```python
from build123d import *

# Parameters (mm, degrees)
ESQUISSE1_W             = 300
ESQUISSE1_H             = 300
BOSS_EXTRU_1_DEPTH      = 12
ESQUISSE2_W             = 250
ESQUISSE2_H             = 250
BOSS_EXTRU_2_DEPTH      = 50
ENL_V_MAT_EXTRU_1_DEPTH = 10
ENL_V_START             = -5
ESQUISSE4_W             = 55
ESQUISSE4_H             = 43.476241007
ENL_V_MAT_EXTRU_2_DEPTH = 5
ESQUISSE6_W             = 240
ESQUISSE6_H             = 240
ENL_V_MAT_EXTRU_3_DEPTH = 50


with BuildPart() as part:
    # Esquisse1 → Boss.-Extru.1 (new body)
    with BuildSketch(Plane.XY):
        Rectangle(ESQUISSE1_W, ESQUISSE1_H)
    extrude(amount=BOSS_EXTRU_1_DEPTH)

    # Esquisse2 → Boss.-Extru.2 (add)
    with BuildSketch(Plane.XY.offset(12)):
        Rectangle(ESQUISSE2_W, ESQUISSE2_H)
    extrude(amount=BOSS_EXTRU_2_DEPTH)

    # Esquisse3 → Enlèv. mat.-Extru.1 (cut)
    with BuildSketch(Plane(origin=(0, 0, 0), x_dir=(-1, 0, 0), z_dir=(0, 0, -1))):
        with BuildLine():
            Line((-15, 92.5), (15, 92.5))
            ThreePointArc((15, 92.5), (27.5, 80), (15, 67.5))
            Line((15, 67.5), (-15, 67.5))
            ThreePointArc((-15, 67.5), (-27.5, 80), (-15, 92.5))
        make_face()
    extrude(amount=-ENL_V_MAT_EXTRU_1_DEPTH, mode=Mode.SUBTRACT)

    # Esquisse4 → Enlèv. mat.-Extru.2 (cut)
    with BuildSketch(Plane(origin=(0, 0, 0), x_dir=(-1, 0, 0), z_dir=(0, 0, -1)).offset(ENL_V_START)):
        with Locations((-0.411034786, 114.238120503)):
            Rectangle(ESQUISSE4_W, ESQUISSE4_H)
    extrude(amount=-ENL_V_MAT_EXTRU_2_DEPTH, mode=Mode.SUBTRACT)

    # Esquisse6 → Enlèv. mat.-Extru.3 (cut)
    with BuildSketch(Plane.XY.offset(62)):
        Rectangle(ESQUISSE6_W, ESQUISSE6_H)
    extrude(amount=-ENL_V_MAT_EXTRU_3_DEPTH, mode=Mode.SUBTRACT)


solid = part.part
```
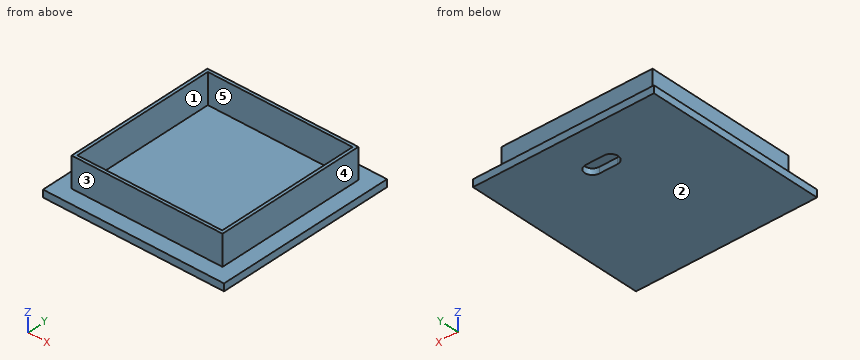
Design review of the part built by this model. Coordinates are the model's own, in mm. Face numbers are marked on the shaded views. A direction names the side the tool comes from. Coordinates: 2 decimals unless noted, no trailing zeros. Order: outer loops, then holes, each group sorted by start corner. A loop starts at its lowest first (then second) coordinate and runs counter-clockwise, first axis right, second up. Notation, with made-up numbers: (23.25, 79) - (71.25, 79) arc R25 ccw to (71.25, 117) - close; hole circle Ø5 at (87.25, 16.25). An arc over 180 degrees is marked (long way). Answer in a Markdown table with one row per item.
(1) Consider section C-C on z = 16. State the section outline as (x, y) points, plus the area to 3 significant figures.
Checked values:
| item | result |
|---|---|
| outline | (-125, -125) - (125, -125) - (125, 125) - (-125, 125) - close; hole (-120, -120) - (120, -120) - (120, 120) - (-120, 120) - close |
| area | 4,900 mm^2 |
(2) Clearance check with flat-ended pins moving along their axes: pin 1 (4 mm diameter, centred on x = -84, z = 47, fed in from -Y); pin 2 (6 mm diameter, centred on x = -31, y = 45, fed in from +Z); pin 3 (15 mm diameter, centred on y = 17, z = 42, fed in from -X). State where each tip first meets the part, or that it passes through.
Checked values:
| item | result |
|---|---|
| pin 1 | y = -125 |
| pin 2 | z = 12 |
| pin 3 | x = -125 |
(3) For the marked faces 4 and 5, list the 3-axis set-ups (+Z, -Z, +X, -X, +Y, -Y) from which the entire face can be reached by the end or side of a thin tool; tool diameter is ignored.
Checked values:
| item | result |
|---|---|
| face 4 | +Z, +X, +Y, -Y |
| face 5 | +Z |
(4) Wall thickness on line 1 along Y through (x, z) = (-93, 26.5); line 2 along Z through (x, y) = (-19.5, 97): over which ranges is each line inside the solid? List them lowest first. Write a range as from..to.
Checked values:
| item | result |
|---|---|
| line 1 | -125..-120, 120..125 |
| line 2 | 0..5, 10..12 |
(5) Consider section D-D on y = 111. State the section outline as (x, z) points, plus the area to 4 significant figures.
Checked values:
| item | result |
|---|---|
| outline | (-150, 0) - (150, 0) - (150, 12) - (125, 12) - (125, 62) - (120, 62) - (120, 12) - (-120, 12) - (-120, 62) - (-125, 62) - (-125, 12) - (-150, 12) - close; hole (-27.09, 5) - (27.91, 5) - (27.91, 10) - (-27.09, 10) - close |
| area | 3,825 mm^2 |
(6) The part is to be moulded in two halves that separate along Y. For the marked faces 1, 2 and 3, say which applies: released by +Y, released by -Y, zero draft, split by the parting line, or undercut.
Checked values:
| item | result |
|---|---|
| face 1 | undercut |
| face 2 | zero draft |
| face 3 | released by -Y |
(7) Consider section B-B on y = 80. State the section outline as (x, z) points, plus the area to 3 significant figures.
Checked values:
| item | result |
|---|---|
| outline | (-150, 0) - (-27.5, 0) - (-27.5, 10) - (27.5, 10) - (27.5, 0) - (150, 0) - (150, 12) - (125, 12) - (125, 62) - (120, 62) - (120, 12) - (-120, 12) - (-120, 62) - (-125, 62) - (-125, 12) - (-150, 12) - close |
| area | 3,550 mm^2 |
(8) Consider section A-A on x = 75. State the section outline as (y, z) points, plus the area to 3 significant figures.
Checked values:
| item | result |
|---|---|
| outline | (-150, 0) - (150, 0) - (150, 12) - (125, 12) - (125, 62) - (120, 62) - (120, 12) - (-120, 12) - (-120, 62) - (-125, 62) - (-125, 12) - (-150, 12) - close |
| area | 4,100 mm^2 |
